Study the drawing (mm; zero at the part's minimum x, y, z) and answer. A direction names the side the tool comes from. Coordinates: 2 decimals unless noted, no trailing zeros. Loops run counter-clockwise (first coordinate to the right, second up) from the corner with the lowest first, then second, coordinate; pieces in that order, holes last. Notation, with made-up numbers: (23.25, 27.5) - (39.25, 27.5) arc R9 ccw to (39.25, 39.5) - close; hole circle Ø3 at (31.5, 82). An arc over 180 degrees is marked (long way). Use one line per item in the form item = value.
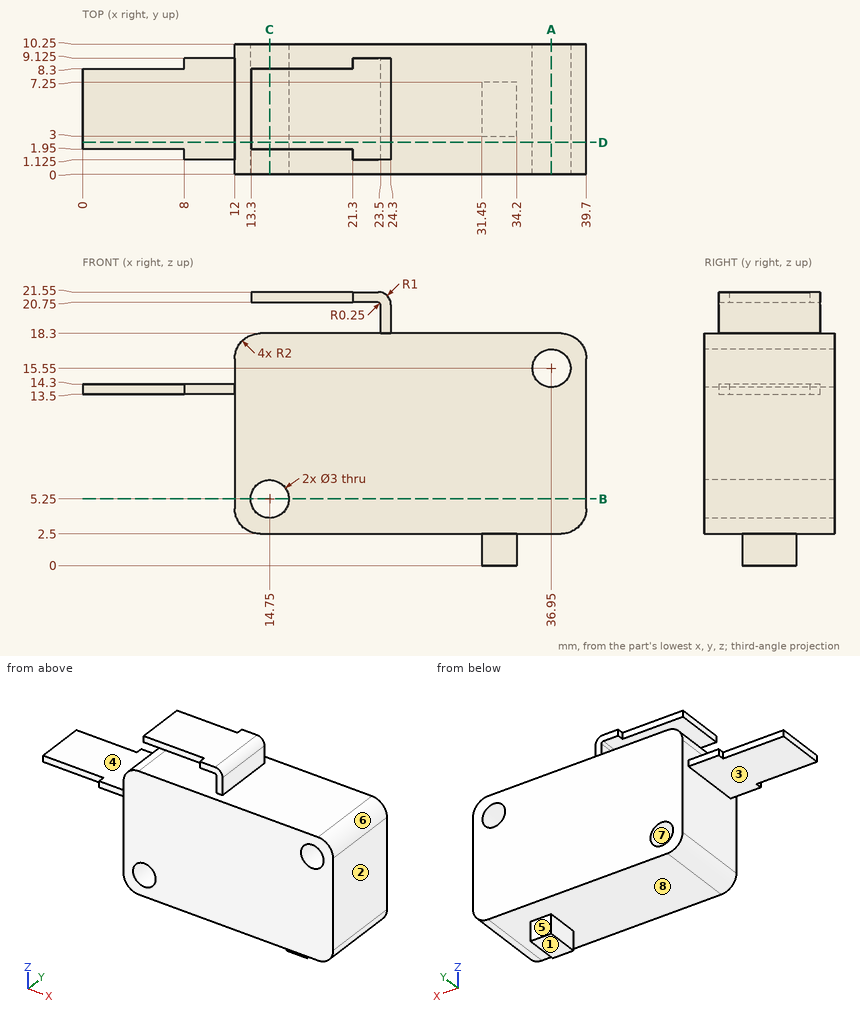
Item 1: Each of these flat-tipped pins is pushed along its axis until it touches: P1, Ø0.8, axis at y = 4.5, z = 1, coming from the -X side; P2, Ø1.1, axis at y = 6, z = 20, coming from the +X side; P3, Ø3, axis at y = 6.5, z = 2.5, coming from the +X side. Where does it stop, or does it pass through?
Results below:
P1 = 31.45
P2 = 24.3
P3 = 39.64
Item 2: Find the intervals of material crossed by L1, parallel to Z at x = 22.5, y = 6.75; L2, parallel to X at y = 3.25, z = 7; L3, parallel to Z at x = 36.95, y = 3, in increasing order.
Results below:
L1 = 2.5 to 18.3, 20.75 to 21.55
L2 = 12 to 39.7
L3 = 2.5 to 14.05, 17.05 to 18.3
Item 3: Which of the six approach directions +Z, -Z, +X, -X, +Y, -Y give full straight-line access (tool end or side, diameter ignored) to the marked faces 1, 2, 3, 4 and 5?
Results below:
face_1 = -Z, +X, -X, +Y, -Y
face_2 = +Z, -Z, +X, +Y, -Y
face_3 = -Z, -X, +Y, -Y
face_4 = +Z, -X, +Y, -Y
face_5 = -Z, +X, -X, +Y
Item 4: The part is cut by section D-D on y = 2.5. Give the vertices of the cut face in (x, z).
Results below:
outline = (0, 13.5) - (12, 13.5) - (12, 4.5) arc R2 ccw to (14, 2.5) - (37.7, 2.5) arc R2 ccw to (39.7, 4.5) - (39.7, 16.3) arc R2 ccw to (37.7, 18.3) - (24.3, 18.3) - (24.3, 20.55) arc R1 ccw to (23.3, 21.55) - (13.3, 21.55) - (13.3, 20.75) - (23.25, 20.75) arc R0.25 cw to (23.5, 20.5) - (23.5, 18.3) - (14, 18.3) arc R2 ccw to (12, 16.3) - (12, 14.3) - (0, 14.3) - close; hole circle Ø3 at (14.75, 5.25); hole circle Ø3 at (36.95, 15.55)
Item 5: The part is cut by section A-A on x = 36.95. Give the vertices of the cut face in (y, z), plus the area to 3 significant figures.
Results below:
outline = (0, 2.5) - (10.25, 2.5) - (10.25, 14.05) - (0, 14.05) - close; (0, 17.05) - (10.25, 17.05) - (10.25, 18.3) - (0, 18.3) - close
area = 131 mm²
Item 6: The part is cut by section C-C on x = 14.75. Give the vertices of the cut face in (y, z), plus the area to 3 significant figures.
Results below:
outline = (0, 2.5) - (10.25, 2.5) - (10.25, 3.75) - (0, 3.75) - close; (0, 6.75) - (10.25, 6.75) - (10.25, 18.3) - (0, 18.3) - close; (1.95, 20.75) - (8.3, 20.75) - (8.3, 21.55) - (1.95, 21.55) - close
area = 136 mm²
Item 7: The part is cut by section B-B on z = 5.25. Give the vertices of the cut face in (x, y), plus the area to 3 significant figures.
Results below:
outline = (12, 0) - (13.25, 0) - (13.25, 10.25) - (12, 10.25) - close; (16.25, 0) - (39.7, 0) - (39.7, 10.25) - (16.25, 10.25) - close
area = 253 mm²
Item 8: For a pull along X with two mould halves and no side action, classify the marked faces 6, 7 and 8 as +X half, -X half, draft (parallel to the pull), parting line (faces both ways), or undercut.
Results below:
face_6 = +X half
face_7 = undercut
face_8 = draft
